For this review, take the finished solid that the model builds, in its own axes (mm). A direction names the side the tool comes from. Round coordinates to 2 decimals unless told otherwise and drop trailing zeros. Write each loop counter-clockwise with the first axis right and the second up, starting at its lowest first coordinate (ties: lowest second). Pieces come first, ordered by that corner, then holes. Notation, with made-up numbers: (3.5, -35.75) -> (59.5, -35.75) arc R31 ccw to (59.5, -8.75) -> close; hole circle Ø1 at (-15.5, -20.5). An arc over 180 degrees is marked (long way). Answer in a Markdown table with one row per item. Add a question column.
Autodesk Inventor part; units mm, degrees
ref_plane "YZ Plane" through (0, 0, 0) normal (1, 0, 0) x (0, 1, 0)
ref_plane "XZ Plane" through (0, 0, 0) normal (0, 1, 0) x (-1, 0, 0)
ref_plane "XY Plane" through (0, 0, 0) normal (0, 0, 1) x (1, 0, 0)
sketch "スケッチ1" plane through (0, 0, 0) normal (0, 0, 1) x (1, 0, 0)
  line L0 (0, 0) -> (0, 17.65)
  line L1 (0, 17.65) -> (28, 17.65)
  line L2 (28, 17.65) -> (28, 30.15)
  line L3 (28, 30.15) -> (58, 30.15)
  line L4 (58, 30.15) -> (58, 0)
  line L5 (58, 0) -> (60, 0)
  line L6 (60, 0) -> (60, 32.15)
  line L7 (60, 32.15) -> (28, 32.15)
  line L8 (28, 32.15) -> (26, 32.15)
  line L9 (26, 32.15) -> (26, 19.65)
  line L10 (26, 19.65) -> (-2, 19.65)
  line L11 (-2, 19.65) -> (-2, 0)
  line L12 (-2, 0) -> (0, 0)
  dimension "d0" = 17.65
  dimension "d1" = 28
  dimension "d2" = 12.5
  dimension "d3" = 30
  dimension "d4" = 2
  dimension "d5" = 32.15
  dimension "d6" = 32
  dimension "d7" = 2
  dimension "d8" = 12.5
  dimension "d9" = 28
extrude "押し出し1" add sketch "スケッチ1" along normal blind 14
sketch "スケッチ2" plane through (60, 0, 0) normal (1, 0, 0) x (0, 0, -1)
  line L0 (0, 0) -> (-14, 0)
  line L1 (-14, 0) -> (0, 0)
  line L2 (0, 0) -> (0, 2)
  line L3 (0, 2) -> (-14, 2)
  line L4 (-14, 2) -> (-14, 0)
  dimension "d12" = 14
  dimension "d13" = 2
extrude "押し出し2" add sketch "スケッチ2" along normal blind 7
sketch "スケッチ3" plane through (-2, 0, 0) normal (-1, 0, 0) x (0, 0, 1)
  line L0 (14, 2) -> (0, 2)
  line L1 (0, 0) -> (14, 0)
  line L2 (14, 0) -> (14, 2)
  line L3 (14, 2) -> (0, 2)
  line L4 (0, 2) -> (0, 0)
  dimension "d16" = 14
extrude "押し出し3" add sketch "スケッチ3" along normal blind 7
sketch "スケッチ4" plane through (0, 0, 14) normal (0, 0, 1) x (1, 0, 0)
  line L0 (60, 32.15) -> (60, 24.15)
  line L1 (60, 24.15) -> (61.6, 24.15)
  arc A0 (61.6, 20.4) -> (61.6, 27.9) centre (61.6, 24.15) ccw
  line L2 (61.6, 24.15) -> (61.6, 20.4) construction
  line L3 (61.6, 24.15) -> (61.6, 27.9) construction
  line L4 (61.6, 27.9) -> (60, 27.9)
  line L5 (61.6, 20.4) -> (60, 20.4)
  line L6 (60, 2) -> (60, 32.15)
  line L7 (60, 27.9) -> (60, 20.4)
  point P0 (0, 0)
  dimension "d47" = 8
  dimension "d48" = 1.6
  dimension "d49" = 3.75
  dimension "d50" = 180
extrude "押し出し4" add sketch "スケッチ4" against normal blind 14
hole "穴3" at (61.6, 24.15, 14) direction (0, 0, -1) diameter 3.75 end through all
sketch "スケッチ7" plane through (0, 0, 14) normal (0, 0, 1) x (1, 0, 0)
  line L0 (60, 32.15) -> (26, 32.15)
  line L1 (26, 32.15) -> (26, 24.15)
  line L2 (26, 24.15) -> (24.4, 24.15)
  arc A0 (24.4, 27.9) -> (24.4, 20.4) centre (24.4, 24.15) ccw
  line L3 (24.4, 27.9) -> (26, 27.9)
  line L4 (24.4, 20.4) -> (26, 20.4)
  line L5 (26, 20.4) -> (26, 27.9)
  line L6 (26, 32.15) -> (26, 19.65)
  circle A1 centre (24.4, 24.15) radius 1.875
  point P0 (0, 0)
  dimension "d60" = 8
  dimension "d61" = 1.6
  dimension "d62" = 3.75
  dimension "d63" = 3.75
extrude "押し出し6" add sketch "スケッチ7" against normal blind 14 contours L1 A1 L5 L4 A0 L3 | L1 L5 A1 picked at (23.6929, 24.15)
hole "穴4" at (24.4, 24.15, 14) direction (0, 0, -1) diameter 3.75 end through all
sketch "スケッチ10" plane through (0, 17.65, 0) normal (0, -1, 0) x (1, 0, 0)
  line L0 (28, 14) -> (58, 14)
  line L1 (0, 0) -> (28, 0)
  line L2 (28, 0) -> (28, 14)
  line L3 (28, 14) -> (0, 14)
  line L4 (0, 14) -> (0, 0)
extrude "押し出し7" cut sketch "スケッチ10" against normal blind 0.6
sketch "スケッチ11" plane through (0, 0, 0) normal (0, -1, 0) x (1, 0, 0)
  line L0 (0, 14) -> (-9, 14)
  line L1 (60, 0) -> (67, 0)
  line L2 (-9, 14) -> (67, 14)
  line L3 (67, 14) -> (67, 0)
  line L4 (67, 0) -> (-9, 0)
  line L5 (-9, 0) -> (-9, 14)
  point P0 (0, 0)
extrude "押し出し8" cut sketch "スケッチ11" against normal blind 0.6
sketch "スケッチ12" plane through (0, 0, 14) normal (0, 0, 1) x (1, 0, 0)
  line L0 (-2, 19.65) -> (-2, 2)
  line L1 (-2, 19.65) -> (4, 19.65)
  line L2 (26, 19.65) -> (-2, 19.65)
  line L3 (4, 19.65) -> (4, 18.25)
  line L4 (0, 18.25) -> (28, 18.25)
  line L5 (4, 18.25) -> (0.2844, 14.5344)
  line L6 (4, 18.25) -> (9.2547, 18.25) construction
  line L7 (0.2844, 14.5344) -> (0, 14.25)
  line L8 (0, 0.6) -> (0, 18.25)
  line L9 (0, 14.25) -> (-2, 14.25)
  line L10 (-2, 14.25) -> (-2, 19.65)
  point P0 (0, 0)
  dimension "d79" = 6
  dimension "d80" = 135
extrude "押し出し9" add sketch "スケッチ12" along normal blind 2
sketch "スケッチ15" plane through (0, 0, 0) normal (0, 0, -1) x (-1, 0, 0)
  line L0 (0, 0.6) -> (0, 18.25)
  line L1 (0, 18.25) -> (-14, 18.25)
  line L2 (-14, 18.25) -> (-14, 0.6)
  line L3 (-14, 0.6) -> (0, 0.6)
  line L4 (0, 0.6) -> (0, 18.25)
  point P0 (0, 0)
  dimension "d88" = 14
extrude "押し出し11" add sketch "スケッチ15" against normal blind 1.4
sketch "スケッチ17" plane through (67, 0, 0) normal (1, 0, 0) x (0, 0, -1)
  line L0 (0, 0.6) -> (-14, 0.6)
  line L1 (0, 0.6) -> (-14, 0.6)
  line L2 (-14, 0.6) -> (-14, 9.5309)
  line L3 (-14, 9.5309) -> (0, 9.5309)
  line L4 (0, 9.5309) -> (0, 0.6)
  point P0 (0, 0)
extrude "押し出し13" cut sketch "スケッチ17" against normal blind 3
sketch "スケッチ18" plane through (-9, 0, 0) normal (-1, 0, 0) x (0, 0, 1)
  line L0 (0, 0.6) -> (14, 0.6)
  line L1 (0, 0.6) -> (14, 0.6)
  line L2 (14, 0.6) -> (14, 6.5)
  line L3 (14, 6.5) -> (0, 6.5)
  line L4 (0, 6.5) -> (0, 0.6)
  point P0 (0, 0)
extrude "押し出し14" cut sketch "スケッチ18" against normal blind 3
hole "穴5" at (-4, 2, 7) direction (0, -1, 0) diameter 2.4 end through all
hole "穴6" at (62, 2, 7) direction (0, -1, 0) diameter 2.4 end through all
mirror "ミラー1" about plane through (31.8158, 20.0509, 0) normal (0, 0, -1) of "押し出し3", "押し出し1", "押し出し4", "穴3", "押し出し2", "穴6", "穴4", "押し出し6", "押し出し7", "押し出し9", "押し出し11", "押し出し14", "押し出し13", "穴5", "押し出し8"
sketch "スケッチ19" plane through (0, 0, 14) normal (0, 0, 1) x (1, 0, 0)
  line L0 (94.8832, 81.412) -> (-62.365, 81.412)
  line L1 (-62.365, 81.412) -> (-62.365, -71.7744)
  line L2 (-62.365, -71.7744) -> (94.8832, -71.7744)
  line L3 (94.8832, -71.7744) -> (94.8832, 81.412)
  point P0 (0, 0)
extrude "押し出し15" cut sketch "スケッチ19" against normal blind 14
sketch "スケッチ20" plane through (-2, 19.65, 14) normal (0, 1, 0) x (1, 0, 0)
  line L0 (17.6833, -4.2941) -> (-12.6138, -4.2941)
  line L1 (-12.6138, -4.2941) -> (-12.6138, 1.0873)
  line L2 (-12.6138, 1.0873) -> (17.6833, 1.0873)
  line L3 (17.6833, 1.0873) -> (17.6833, -4.2941)
  point P0 (2, 14)
extrude "押し出し16" cut sketch "スケッチ20" against normal blind 14
sketch "スケッチ21" plane through (26, 27.9, -14) normal (-1, 0, 0) x (0, 0, 1)
  line L0 (0, -8.25) -> (-2, -8.25)
  line L1 (-2, -8.25) -> (18.9234, -8.25)
  line L2 (18.9234, -8.25) -> (18.9234, 5.2405)
  line L3 (18.9234, 5.2405) -> (-2, 5.2405)
  line L4 (-2, 5.2405) -> (-2, -8.25)
  point P0 (14, -27.9)
split body "分割1" sketch "スケッチ21" result one side removed curves L2 L3 L4 L1 removed pieces at (9.3333, 19.15, -4.6667) (58.5, 13.3, -4.6667)
properties part number "センサ冶具小"
1. We need section A-A (y = 24.15). Write out the cut boundary in (x, z) (3 decimals).
2. Clearance check with flat-ended pins moving along their axes: pin 1 Ø3 at (x, y) = (45, 30) entering from -Z; pin 2 Ø1.5 at (y, z) = (30.5, -4.5) entering from -X; pin 3 Ø1.3 at (x, z) = (25, -8.5) entering from -Y; pin 4 Ø0.8 at (x, z) = (25, -5.5) entering from +Y. State where each tip first meets the part, or that it passes through.
3. The part is to be moulded in two halves that separate along X. For faces 1 (the flat face through (43, 31, -14)), 2 (the cylindrical face through (24.482, 26.023, -6.902)), 3 (the flat face through (43, 30.15, -7)), 4 (the flat face through (60, 30, -7)), say which applies: pulls with the +X half, pulls with the -X half, needs draft (parallel to the pull), parting line crosses it, or undercut.
4. We need section B-B (z = -3.5). Write out the cut boundary in (x, y) (3 decimals), plus the area to 3 significant figures.
5. For L1, parallel to X at y = 24.15, z = -4 (3 decimals); L2, parallel to Y at x = 61.6, z = -8 (3 decimals); L3, parallel to Y at x = 45, z = -4, list the stretches that pass through material, from the lowest coordinate up. Write a range as [from, to].
6. We need section C-C (y = 29). Write out the cut boundary in (x, z), plus the area to 3 significant figures.
7. Tool access review of faces 5 (the flat face through (25, 20.4, -7)), 6 (the flat face through (28, 25, -7)), 7 (the flat face through (25, 27.9, -7)), 8 (the flat face through (61, 27.9, -7)): name each direction out of +Z, -Z, +X, -X, +Y, -Y from which nothing blocks a thin tool from reaching the whole face with its end or side.
8. We need section D-D (x = 61). Write out the cut boundary in (y, z).
Response:
| question | item | result |
|---|---|---|
| 1 | outline | (20.65, -14) -> (22.525, -14) -> (22.525, 0) -> (20.65, 0) -> close; (26.275, -14) -> (28, -14) -> (28, 0) -> (26.275, 0) -> close; (58, -14) -> (59.725, -14) -> (59.725, 0) -> (58, 0) -> close; (63.475, -14) -> (65.35, -14) -> (65.35, 0) -> (63.475, 0) -> close |
| 2 | pin 1 | z = -14 |
| 2 | pin 2 | x = 26 |
| 2 | pin 3 | y = 20.4 |
| 2 | pin 4 | y = 27.9 |
| 3 | face 1 | needs draft |
| 3 | face 2 | undercut |
| 3 | face 3 | undercut |
| 3 | face 4 | pulls with the +X half |
| 4 | outline | (24.4, 20.4) -> (26, 20.4) -> (26, 19.65) -> (28, 19.65) -> (28, 30.15) -> (58, 30.15) -> (58, 19.65) -> (60, 19.65) -> (60, 20.4) -> (61.6, 20.4) arc R3.75 ccw to (61.6, 27.9) -> (60, 27.9) -> (60, 32.15) -> (26, 32.15) -> (26, 27.9) -> (24.4, 27.9) arc R3.75 ccw to start; hole circle Ø3.75 at (24.4, 24.15); hole circle Ø3.75 at (61.6, 24.15) |
| 4 | area | 156 mm2 |
| 5 | L1 | [20.65, 22.525], [26.275, 28], [58, 59.725], [63.475, 65.35] |
| 5 | L2 | [20.4, 22.275], [26.025, 27.9] |
| 5 | L3 | [30.15, 32.15] |
| 6 | outline | (26, -14) -> (28, -14) -> (28, 0) -> (26, 0) -> close; (58, -14) -> (60, -14) -> (60, 0) -> (58, 0) -> close |
| 6 | area | 56.0 mm2 |
| 7 | face 5 | +Z, -Z, -X, -Y |
| 7 | face 6 | +Z, -Z, -Y |
| 7 | face 7 | +Z, -Z, -X, +Y |
| 7 | face 8 | +Z, -Z, +X, +Y |
| 8 | outline | (20.4, -14) -> (22.37, -14) -> (22.37, 0) -> (20.4, 0) -> close; (25.93, -14) -> (27.9, -14) -> (27.9, 0) -> (25.93, 0) -> close |
